The listing builds one solid part. Answer for the finished solid, in the listing's coordinates (mm). A direction names the side the tool comes from. Coordinates: 2 decimals unless noted, no trailing zeros. Order: outer loops, then holes, each group sorted by start corner. A loop starts at its lowest first (then second) coordinate and runs counter-clockwise, first axis right, second up. Notation, with made-up numbers: (17.25, 55.25) -> (31.25, 55.25) arc R27 ccw to (31.25, 80.25) -> close; hole circle Ø4 at (89.5, 85). An arc over 180 degrees is marked (long way). Return JSON: item names as keys, results as strings.
```python
from build123d import *

# Parameters (mm, degrees)
F0_W     = 30
F0_H     = 12
F0_W_2   = 19
F1_DEPTH = 3.8
F2_W     = 1.9557817429
F2_H     = 2.5
F2_W_2   = 17.5
F2_H_2   = 2
F2_W_3   = 2
F2_W_4   = 16.5
F2_W_5   = 4.5
F2_W_6   = 2.5
F2_W_7   = 2.0442182571
F3_DEPTH = 25
F4_DEPTH = 1
F2_H_3   = 2.75
F2_H_4   = 2.25
F2_H_5   = 4.75
F2_H_6   = 0.25
F5_DEPTH = 2
F6_W     = 21
F6_H     = 5
F6_R     = 1
F7_DEPTH = 1
F8_DEPTH = 2
F9_R     = 0.99999


# Not quite as in the source:
# - a fillet or chamfer is up to 0.001 mm smaller than in the source, because OpenCascade refuses the exact size


with BuildPart() as f1:
    # F0 (on Top) → F1 (new body)
    with BuildSketch(Plane.XY):
        with Locations((15, -6)):
            Rectangle(F0_W, F0_H)
        with Locations((-9.5, -6)):
            Rectangle(F0_W_2, F0_H)
    extrude(amount=F1_DEPTH)

    # F2 (on face) → F3 (cut)
    with BuildSketch(Plane.XY.offset(3.8)):
        with Locations((-18.0221091285, -6)):
            Rectangle(F2_W, F2_H)
        with Locations((-6.25, -3.75)):
            Rectangle(F2_W_2, F2_H_2)
        with Locations((-6.25, -6)):
            Rectangle(F2_W_2, F2_H)
        with Locations((-6.25, -8.5)):
            Rectangle(F2_W_2, F2_H)
        with Locations((3.5, -3.75)):
            Rectangle(F2_W_3, F2_H_2)
        with Locations((3.5, -6)):
            Rectangle(F2_W_3, F2_H)
        with Locations((3.5, -8.5)):
            Rectangle(F2_W_3, F2_H)
        with Locations((12.75, -8.5)):
            Rectangle(F2_W_4, F2_H)
        with Locations((12.75, -6)):
            Rectangle(F2_W_4, F2_H)
        with Locations((12.75, -3.75)):
            Rectangle(F2_W_4, F2_H_2)
        with Locations((23.25, -6)):
            Rectangle(F2_W_5, F2_H)
        with Locations((26.5, -6)):
            Rectangle(F2_W_3, F2_H)
        with Locations((28.75, -6)):
            Rectangle(F2_W_6, F2_H)
        Polygon((19, -12), (30, -12), (30, -10), (27.5, -10), (25.5, -10), (19, -10), align=None)
        with Locations((-16.0221091285, -6)):
            Rectangle(F2_W_7, F2_H)
    extrude(amount=-F3_DEPTH, mode=Mode.SUBTRACT)

    # F2 (on face) → F4 (join)
    with BuildSketch(Plane.XY.offset(3.8)):
        with Locations((-18.0221091285, -6)):
            Rectangle(F2_W, F2_H)
        with Locations((23.25, -6)):
            Rectangle(F2_W_5, F2_H)
        with Locations((26.5, -6)):
            Rectangle(F2_W_3, F2_H)
        with Locations((28.75, -6)):
            Rectangle(F2_W_6, F2_H)
        with Locations((-16.0221091285, -6)):
            Rectangle(F2_W_7, F2_H)
    extrude(amount=-F4_DEPTH)

    # F2 (on face) → F5 (join)
    with BuildSketch(Plane.XY.offset(3.8)):
        with Locations((3.5, -1.375)):
            Rectangle(F2_W_3, F2_H_3)
        with Locations((3.5, -3.75)):
            Rectangle(F2_W_3, F2_H_2)
        with Locations((3.5, -6)):
            Rectangle(F2_W_3, F2_H)
        with Locations((3.5, -8.5)):
            Rectangle(F2_W_3, F2_H)
        with Locations((3.5, -10.875)):
            Rectangle(F2_W_3, F2_H_4)
        with Locations((26.5, -2.375)):
            Rectangle(F2_W_3, F2_H_5)
        with Locations((26.5, -6)):
            Rectangle(F2_W_3, F2_H)
        with Locations((26.5, -8.5)):
            Rectangle(F2_W_3, F2_H)
        with Locations((26.5, -9.875)):
            Rectangle(F2_W_3, F2_H_6)
    extrude(amount=F5_DEPTH)

    # F6 (on face) → F7 (join)
    with BuildSketch(Plane.XY.offset(5.8)):
        with Locations((15, -6.5)):
            Rectangle(F6_W, F6_H)
        with Locations((12.75, -6.5)):
            Circle(F6_R, mode=Mode.SUBTRACT)
    extrude(amount=-F7_DEPTH)

    # F6 (on face) → F8 (join)
    with BuildSketch(Plane.XY.offset(5.8)):
        with Locations((12.75, -6.5)):
            Circle(F6_R)
    extrude(amount=-F8_DEPTH)

    # F9 (radius 1 in the source; OpenCascade refuses exactly that, so slightly less here)
    f9_edges = [f1.edges().sort_by_distance(p)[0] for p in [
        (11.75, -6.5, 3.8),
        (25.5, -6.5, 4.8),
        (4.5, -6.5, 4.8),
        (4.5, -10.875, 3.8),
        (4.5, -1.375, 3.8),
    ]]
    fillet(f9_edges, radius=F9_R)


solid = f1.part
```
Item 1: Determine the mould class of faces 1 (the flat face through (27.5, -5, 5)), 2 (the flat face through (-15, -6, 3)), 3 (the flat face through (25, -6, 2.8)) for opening direction X: pulls with the +X half, pulls with the -X half, needs draft (parallel to the pull), parting line crosses it, or undercut.
Answer list:
{"face 1": "pulls with the +X half", "face 2": "undercut", "face 3": "needs draft"}
Item 2: The part is cut by section C-C on z = 1. Determine the outline of the cut face in (x, y), plus the area to 4 significant figures.
Answer list:
{"outline": "(-19, -12) -> (19, -12) -> (19, -10) -> (30, -10) -> (30, -7.25) -> (21, -7.25) -> (21, -9.75) -> (-15, -9.75) -> (-15, -7.25) -> (-19, -7.25) -> close; (-19, -4.75) -> (-15, -4.75) -> (-15, -2.75) -> (21, -2.75) -> (21, -4.75) -> (30, -4.75) -> (30, 0) -> (-19, 0) -> close", "area": "281.5 mm2"}
Item 3: The part is cut by section A-A on x = -8.5. Determine the outline of the cut face in (y, z), plus the area to 3 significant figures.
Answer list:
{"outline": "(-12, 0) -> (-9.75, 0) -> (-9.75, 3.8) -> (-12, 3.8) -> close; (-2.75, 0) -> (0, 0) -> (0, 3.8) -> (-2.75, 3.8) -> close", "area": "19.0 mm2"}
Item 4: Flat-ended cylindrical pins translate along their axes: pin 1 (1 mm diameter, centred on x = 16.5, z = 5, fed in from +Y); pin 2 (5.5 mm diameter, centred on x = 19, y = -6, fed in from -Z); pin 3 (1 mm diameter, centred on x = 11.5, y = -7.5, fed in from -Z); pin 4 (0.8 mm diameter, centred on x = 25.5, y = -6, fed in from -Z). Find the tip coordinate at first contact, or state that the pin passes through.
Answer list:
{"pin 1": "y = -4", "pin 2": "z = 0", "pin 3": "z = 4.8", "pin 4": "z = 2.8"}
Item 5: Which of the six approach directions +Z, -Z, +X, -X, +Y, -Y give full straight-line access (tool end or side, diameter ignored) to faces 4 (the flat face through (-11, -2, 3.8)), 5 (the cylindrical face through (4.801, -6.465, 4.515)), 6 (the flat face through (5, 0, 2)), 7 (the flat face through (4.5, -3.8, 5.2)), 8 (the flat face through (19, -11, 2))?
Answer list:
{"face 4": "+Z, -X, +Y, -Y", "face 5": "-Z", "face 6": "+Z, -Z, +X, -X, +Y", "face 7": "+Z", "face 8": "+Z, -Z, +X, -Y"}
Item 6: Find the intervals of material crossed by probe 1 along Y at (x, z) = (-13, 2.05); probe 2 along X at (y, z) = (-3, 0.6), in increasing order.
Answer list:
{"probe 1": "-12 to -9.75, -2.75 to 0", "probe 2": "-19 to -15, 21 to 30"}
Item 7: The part is cut by section B-B on x = 18.5. Determine the outline of the cut face in (y, z).
Answer list:
{"outline": "(-12, 0) -> (-9.75, 0) -> (-9.75, 3.8) -> (-12, 3.8) -> close; (-9, 4.8) -> (-4, 4.8) -> (-4, 5.8) -> (-9, 5.8) -> close; (-2.75, 0) -> (0, 0) -> (0, 3.8) -> (-2.75, 3.8) -> close"}
Item 8: The part is cut by section D-D on y = -0.75. Determine the outline of the cut face in (x, z).
Answer list:
{"outline": "(-19, 0) -> (30, 0) -> (30, 3.8) -> (27.5, 3.8) -> (27.5, 5.8) -> (25.5, 5.8) -> (25.5, 3.8) -> (5.5, 3.8) arc R1 cw to (4.5, 4.8) -> (4.5, 5.8) -> (2.5, 5.8) -> (2.5, 3.8) -> (-19, 3.8) -> close"}
